The model under review builds one solid part; all positions refer to its coordinate system, in mm. A direction names the side the tool comes from. Coordinates: 2 decimals unless noted, no trailing zeros. Loops run counter-clockwise (first coordinate to the right, second up) from the corner with the lowest first, then second, coordinate; pieces in that order, holes last. Notation, with made-up numbers: (-28.5, 27) - (7.5, 27) arc R24 ccw to (7.5, 42) - close; hole circle Ø4 at (58, -22.75). An arc over 180 degrees is marked (long way). One line per item, written item: value. Start each with the question number.
1. We need section C-C, the plane x = 0. Give the boundary of the cut face in (y, z).
2. For faces 1 (the face through (-50, 1, -1)), 2 (the face through (-27, -4, 0)), 3 (the face through (27, 4, 0)), list the 3-axis set-ups (+Z, -Z, +X, -X, +Y, -Y) from which the entire face can be reached by the end or side of a thin tool; tool diameter is ignored.
3. Insertion check: P1, Ø9, axis at x = 53.74, y = 0, coming from the +Z side; P2, Ø1.5, axis at y = -2, z = -2, coming from the -X side; P3, Ø2, axis at x = 32.5, z = -0.5, coming from the +Y side. Each pin has a flat end and moves straight along its axis. Give the tip position at first contact, or say it passes through.
4. To check wall thickness, follow line 1 (X direction, y = 2.25, z = -1.75); line 2 (X direction, y = 6.25, z = -3.5); line 3 (X direction, y = -1, z = -2.25). State the ranges of each line that lie inside material, in increasing order.
5. We need section A-A, the plane z = -2. Give the boundary of the cut face in (x, y), then the cut area to 3 significant figures.
6. We need section B-B, the plane y = 0. Give the boundary of the cut face in (x, z), then the cut area to 3 significant figures.
from build123d import *

# Parameters (mm, degrees)
SKETCH1_W           = 120
SKETCH1_H           = 8
SKETCH1_R           = 1.5
BOSS_EXTRUDE1_DEPTH = 3
FILLET2_R           = 4
FILLET3_R           = 4
FILLET4_R           = 4
SKETCH2_R           = 1.5
CUT_EXTRUDE1_DEPTH  = 3
CUT_EXTRUDE2_DEPTH  = 3
SKETCH4_R           = 1.5
BOSS_EXTRUDE2_DEPTH = 4
SKETCH5_R           = 7.5
SKETCH5_R_2         = 1.5
BOSS_EXTRUDE3_DEPTH = 7
SKETCH6_R           = 5
CUT_EXTRUDE3_DEPTH  = 4
SKETCH7_R           = 3.5
CUT_EXTRUDE4_DEPTH  = 4
SKETCH8_R           = 5.1
SKETCH8_R_2         = 5
CUT_EXTRUDE5_DEPTH  = 4


with BuildPart() as part:
    # Sketch1 → Boss-Extrude1 (new body)
    with BuildSketch(Plane.XY):
        Rectangle(SKETCH1_W, SKETCH1_H)
        Circle(SKETCH1_R, mode=Mode.SUBTRACT)
    extrude(amount=BOSS_EXTRUDE1_DEPTH)

    # Fillet2
    fillet2_edges = [part.edges().sort_by_distance(p)[0] for p in [
        (-60, 4, 1.5),
    ]]
    fillet(fillet2_edges, radius=FILLET2_R)

    # Fillet3
    fillet3_edges = [part.edges().sort_by_distance(p)[0] for p in [
        (-60, -4, 1.5),
    ]]
    fillet(fillet3_edges, radius=FILLET3_R - 0.0001)  # a hair under: the kernel refuses the full size

    # Fillet4
    fillet4_edges = [part.edges().sort_by_distance(p)[0] for p in [
        (60, -4, 1.5),
        (60, 4, 1.5),
    ]]
    fillet(fillet4_edges, radius=FILLET4_R - 0.0001)  # a hair under: the kernel refuses the full size

    # Sketch2 → Cut-Extrude1 (cut)
    with BuildSketch(Plane.XY.offset(3)):
        with Locations((-53.738621028, 0)):
            Circle(SKETCH2_R)
        with Locations((53.738621028, 0)):
            Circle(SKETCH2_R)
    extrude(amount=-CUT_EXTRUDE1_DEPTH, mode=Mode.SUBTRACT)

    # Sketch3 → Cut-Extrude2 (cut)
    with BuildSketch(Plane.XY.offset(3)):
        with BuildLine():
            ThreePointArc((-53.738621028, -4), (-57.738621028, 0), (-53.738621028, 4))
            Line((-53.738621028, 4), (-56, 4))
            ThreePointArc((-56, 4), (-58.828427125, 2.828427125), (-60, 0))
            ThreePointArc((-60, 0), (-58.828427125, -2.828427125), (-56, -4))
            Line((-56, -4), (-53.738621028, -4))
        make_face()
        with BuildLine():
            ThreePointArc((60, 0), (58.828427125, 2.828427125), (56, 4))
            Line((56, 4), (53.738621028, 4))
            ThreePointArc((53.738621028, 4), (57.738621028, 0), (53.738621028, -4))
            Line((53.738621028, -4), (56, -4))
            ThreePointArc((56, -4), (58.828427125, -2.828427125), (60, 0))
        make_face()
    extrude(amount=-CUT_EXTRUDE2_DEPTH, mode=Mode.SUBTRACT)


with BuildPart() as cut_extrude2_kept_piece:
    # of the separate pieces the step leaves, the one the design keeps (cut_extrude2_pieces_kept)
    add(part.part.solids().sort_by_distance((-53.738621028, -4, 0))[0])

    # Sketch4 → Boss-Extrude2 (add)
    with BuildSketch(Plane(origin=(0, 0, 0), x_dir=(-1, 0, 0), z_dir=(0, 0, -1))):
        with BuildLine():
            Line((53.738621028, 4), (-53.738621028, 4))
            ThreePointArc((-53.738621028, 4), (-57.738621028, 0), (-53.738621028, -4))
            Line((-53.738621028, -4), (53.738621028, -4))
            ThreePointArc((53.738621028, -4), (57.738621028, 0), (53.738621028, 4))
        make_face()
        with Locations(Location((-53.738621028, 0, 0), (0, 0, 180))):
            Circle(SKETCH4_R, mode=Mode.SUBTRACT)
        Circle(SKETCH4_R, mode=Mode.SUBTRACT)
        with Locations(Location((53.738621028, 0, 0), (0, 0, 180))):
            Circle(SKETCH4_R, mode=Mode.SUBTRACT)
    extrude(amount=BOSS_EXTRUDE2_DEPTH)

    # Sketch5 → Boss-Extrude3 (add, through all)
    # profile 1 of 3: a face of its own
    with BuildSketch(Plane.XY.offset(3)):
        with Locations((-53.738621028, 0)):
            Circle(SKETCH5_R)
        with Locations((-53.738621028, 0)):
            Circle(SKETCH5_R_2, mode=Mode.SUBTRACT)
    # profile 2 of 3: a face of its own
    with BuildSketch(Plane.XY.offset(3)):
        Circle(SKETCH5_R)
        with Locations(Location((0, 0, 0), (0, 0, 180))):
            Circle(SKETCH5_R_2, mode=Mode.SUBTRACT)
    # profile 3 of 3: a face of its own
    with BuildSketch(Plane.XY.offset(3)):
        with Locations((53.738621028, 0)):
            Circle(SKETCH5_R)
        with Locations((53.738621028, 0)):
            Circle(SKETCH5_R_2, mode=Mode.SUBTRACT)
    extrude(amount=-BOSS_EXTRUDE3_DEPTH)

    # Sketch6 → Cut-Extrude3 (cut)
    with BuildSketch(Plane.XY.offset(3)):
        with Locations((-53.738621028, 0)):
            Circle(SKETCH6_R)
        Circle(SKETCH6_R)
        with Locations((53.738621028, 0)):
            Circle(SKETCH6_R)
    extrude(amount=-CUT_EXTRUDE3_DEPTH, mode=Mode.SUBTRACT)

    # Sketch7 → Cut-Extrude4 (cut)
    with BuildSketch(Plane(origin=(0, 0, -4), x_dir=(-1, 0, 0), z_dir=(0, 0, -1))):
        with Locations((-53.738621028, 0)):
            Circle(SKETCH7_R)
        Circle(SKETCH7_R)
        with Locations((53.738621028, 0)):
            Circle(SKETCH7_R)
    extrude(amount=-CUT_EXTRUDE4_DEPTH, mode=Mode.SUBTRACT)

    # Sketch8 → Cut-Extrude5 (cut)
    # profile 1 of 3: a face of its own
    with BuildSketch(Plane.XY.offset(3)):
        with Locations((-53.738621028, 0)):
            Circle(SKETCH8_R)
        with Locations((-53.738621028, 0)):
            Circle(SKETCH8_R_2, mode=Mode.SUBTRACT)
    # profile 2 of 3: a face of its own
    with BuildSketch(Plane.XY.offset(3)):
        Circle(SKETCH8_R)
        Circle(SKETCH8_R_2, mode=Mode.SUBTRACT)
    # profile 3 of 3: a face of its own
    with BuildSketch(Plane.XY.offset(3)):
        with Locations((53.738621028, 0)):
            Circle(SKETCH8_R)
        with Locations((53.738621028, 0)):
            Circle(SKETCH8_R_2, mode=Mode.SUBTRACT)
    extrude(amount=-CUT_EXTRUDE5_DEPTH, mode=Mode.SUBTRACT)


solid = cut_extrude2_kept_piece.part
Findings below:
1. outline: (-7.5, -4) - (-3.5, -4) - (-3.5, -1) - (-5.1, -1) - (-5.1, 3) - (-7.5, 3) - close; (3.5, -4) - (7.5, -4) - (7.5, 3) - (5.1, 3) - (5.1, -1) - (3.5, -1) - close
2. face 1: +Z
2. face 2: +Z, -Z, -Y
2. face 3: +Z, -Z, +Y
3. P1: z = -1
3. P2: x = -61.13
3. P3: y = 4
4. line 1: -60.89 to -56.42, -51.06 to -2.68, 2.68 to 51.06, 56.42 to 60.89
4. line 2: -57.88 to -49.59, -4.15 to 4.15, 49.59 to 57.88
4. line 3: -61.17 to -57.09, -50.38 to -3.35, 3.35 to 50.38, 57.09 to 61.17
5. outline: (-47.39, -4) - (-6.34, -4) arc R7.5 ccw to (6.34, -4) - (47.39, -4) arc R7.5 ccw (long way) to (47.39, 4) - (6.34, 4) arc R7.5 ccw to (-6.34, 4) - (-47.39, 4) arc R7.5 ccw (long way) to start; hole circle Ø7 at (-53.74, 0); hole circle Ø7 at (0, 0); hole circle Ø7 at (53.74, 0)
5. area: 1,050 mm2
6. outline: (-61.24, -4) - (-57.24, -4) - (-57.24, -1) - (-58.84, -1) - (-58.84, 3) - (-61.24, 3) - close; (-50.24, -4) - (-3.5, -4) - (-3.5, -1) - (-5.1, -1) - (-5.1, 3) - (-48.64, 3) - (-48.64, -1) - (-50.24, -1) - close; (3.5, -4) - (50.24, -4) - (50.24, -1) - (48.64, -1) - (48.64, 3) - (5.1, 3) - (5.1, -1) - (3.5, -1) - close; (57.24, -4) - (61.24, -4) - (61.24, 3) - (58.84, 3) - (58.84, -1) - (57.24, -1) - close
6. area: 672 mm2
